Geometry: final body of the model. Coordinates: model frame, mm. Face numbers are marked on the shaded views. A direction names the side the tool comes from. Round coordinates to 2 decimals unless told otherwise and drop trailing zeros. Loops run counter-clockwise (first coordinate to the right, second up) from the corner with the lowest first, then second, coordinate; pieces in that order, holes last. Notation, with made-up numbers: M -11.5,81.5 L 33.5,81.5 A16 ccw 33.5,89.5 Z; hole C 2.5,3 d7. An arc over 180 degrees is marked long. Return JSON: item names as keys, results as strings.
from build123d import *

# Parameters (mm, degrees)
SKETCH_1_R          = 2
EXTRUDE_1_DEPTH     = 20
CUT_EXTRUDE_2_DEPTH = 14


with BuildPart() as part:
    # 草图1 → 凸台-拉伸1 (new body)
    with BuildSketch(Plane.XY):
        with BuildLine():
            Line((8.641852584, -30.917005362), (23.544151188, -8.402088166))
            Line((23.544151188, -8.402088166), (13.777542747, 27.154145307))
            ThreePointArc((13.777542747, 27.154145307), (13.313905715, 28.119907916), (12.540501442, 28.861192305))
            Line((12.540501442, 28.861192305), (8.156572048, 31.762851872))
            ThreePointArc((8.156572048, 31.762851872), (5.902657289, 32.20096852), (3.999103626, 30.917005362))
            Line((3.999103626, 30.917005362), (-23.045808654, -9.94339992))
            ThreePointArc((-23.045808654, -9.94339992), (-23.483925302, -12.197314679), (-22.199962144, -14.100868342))
            Line((-22.199962144, -14.100868342), (4.484384162, -31.762851872))
            ThreePointArc((4.484384162, -31.762851872), (6.738298922, -32.20096852), (8.641852584, -30.917005362))
        make_face()
        with Locations((6.410183267, -27.041485776)):
            Circle(SKETCH_1_R, mode=Mode.SUBTRACT)
        with Locations((17.448922973, -10.363769335)):
            Circle(SKETCH_1_R, mode=Mode.SUBTRACT)
        with Locations((-18.606391395, -10.483376217)):
            Circle(SKETCH_1_R, mode=Mode.SUBTRACT)
        with Locations((-7.567651689, 6.194340225)):
            Circle(SKETCH_1_R, mode=Mode.SUBTRACT)
        with BuildLine():
            Line((3.614616276, -20.394320576), (9.685923114, -11.221576533))
            ThreePointArc((9.685923114, -11.221576533), (9.978000879, -9.718966694), (9.122025441, -8.449930919))
            Line((9.122025441, -8.449930919), (-4.220147712, 0.381060846))
            ThreePointArc((-4.220147712, 0.381060846), (-5.722757552, 0.673138612), (-6.991793327, -0.182836827))
            Line((-6.991793327, -0.182836827), (-13.063100166, -9.35558087))
            ThreePointArc((-13.063100166, -9.35558087), (-13.355177931, -10.858190709), (-12.499202492, -12.127226485))
            Line((-12.499202492, -12.127226485), (0.842970661, -20.95821825))
            ThreePointArc((0.842970661, -20.95821825), (2.3455805, -21.250296015), (3.614616276, -20.394320576))
        make_face(mode=Mode.SUBTRACT)
        with BuildLine():
            Line((-2.181398369, 8.62528164), (12.553966944, -1.1278439))
            ThreePointArc((12.553966944, -1.1278439), (14.831422966, -1.079549075), (15.586409089, 1.069668056))
            Line((15.586409089, 1.069668056), (9.371464219, 23.695744666))
            ThreePointArc((9.371464219, 23.695744666), (7.758191259, 25.140995222), (5.775124401, 24.269878325))
            Line((5.775124401, 24.269878325), (-2.745296043, 11.396927255))
            ThreePointArc((-2.745296043, 11.396927255), (-3.037373808, 9.894317415), (-2.181398369, 8.62528164))
        make_face(mode=Mode.SUBTRACT)
    extrude(amount=EXTRUDE_1_DEPTH)

    # 草图2 → 切除-拉伸2 (cut)
    with BuildSketch(Plane.XY.offset(20)):
        Polygon((23.544151188, -8.402088166), (-8.143510051, 12.571517276), (4.702402911, 35.561922015), (37.191732114, 19.156948223), align=None)
    extrude(amount=-CUT_EXTRUDE_2_DEPTH, mode=Mode.SUBTRACT)


solid = part.part
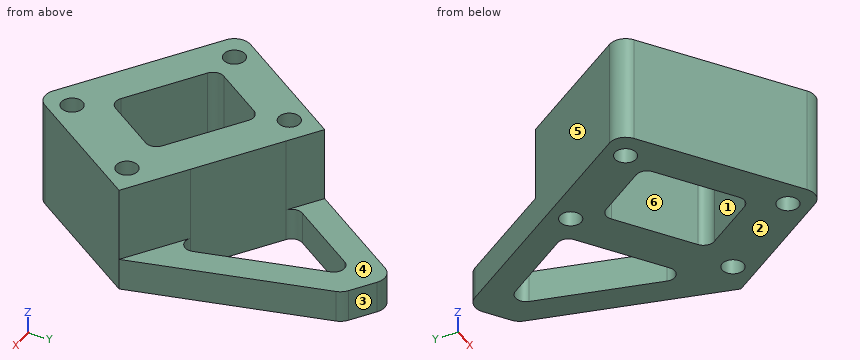
Q1. Section query C-C (z = 1.5). Output: boundary loops of the cut face in (x, y), plus the area to 3 significant figures.
Determined:
{"outline": "M -23.05,-9.94 A3 ccw -22.2,-14.1 L 4.48,-31.76 A3 ccw 8.64,-30.92 L 23.54,-8.4 L 13.78,27.15 A3 ccw 12.54,28.86 L 8.16,31.76 A3 ccw 4,30.92 Z; hole C -18.61,-10.48 d4; hole M -13.06,-9.36 A2 ccw -12.5,-12.13 L 0.84,-20.96 A2 ccw 3.61,-20.39 L 9.69,-11.22 A2 ccw 9.12,-8.45 L -4.22,0.38 A2 ccw -6.99,-0.18 Z; hole C -7.57,6.19 d4; hole M -2.75,11.4 A2 ccw -2.18,8.63 L 12.55,-1.13 A2 ccw 15.59,1.07 L 9.37,23.7 A2 ccw 5.78,24.27 Z; hole C 6.41,-27.04 d4; hole C 17.45,-10.36 d4", "area": "1,120 mm^2"}
Q2. Pull-direction query (X, two-part tool) for the marked faces 1, 2 and 3; classes: pulls with the +X half, pulls with the -X half, needs draft (parallel to the pull), parting line crosses it, or undercut.
Determined:
{"face 1": "undercut", "face 2": "needs draft", "face 3": "pulls with the +X half"}
Q3. Section query A-A (x = -11.5). Output: boundary loops of the cut face in (y, z), plus the area to 3 significant figures.
Determined:
{"outline": "M -21.18,0 L -12.79,0 L -12.79,20 L -21.18,20 Z; M -6.99,0 L 7.5,0 L 7.5,20 L -6.99,20 Z", "area": "458 mm^2"}
Q4. Section query D-D (z = 15.25). Output: boundary loops of the cut face in (x, y).
Determined:
{"outline": "M -23.05,-9.94 A3 ccw -22.2,-14.1 L 4.48,-31.76 A3 ccw 8.64,-30.92 L 23.54,-8.4 L -8.14,12.57 Z; hole C -18.61,-10.48 d4; hole M -13.06,-9.36 A2 ccw -12.5,-12.13 L 0.84,-20.96 A2 ccw 3.61,-20.39 L 9.69,-11.22 A2 ccw 9.12,-8.45 L -4.22,0.38 A2 ccw -6.99,-0.18 Z; hole C -7.57,6.19 d4; hole C 6.41,-27.04 d4; hole C 17.45,-10.36 d4"}
Q5. Pin query (flat end, axial travel): pin 1 (2 mm diameter, centred on x = 1, z = 10.5, fed in from -Y); pin 2 (1.5 mm diameter, centred on y = 4, z = 14, fed in from +X); pin 3 (4 mm diameter, centred on y = -17.5, z = 9, fed in from -X). Return the tip coordinate at first contact, or that it passes through.
Determined:
{"pin 1": "stops at y = -30.12", "pin 2": "stops at x = 5.94", "pin 3": "stops at x = -20.09"}
Q6. Material intervals for L1, parallel to Y at x = 3, z = 4.5; L2, parallel to Y at x = 5, z = 5.75; L3, parallel to X at y = 6.5, z = 5.75, sorted ascending.
Determined:
{"L1": "y = -30.78 to -20.99, -4.4 to 5.2, 20.08 to 29.41", "L2": "y = -32.04 to -28.46, -25.62 to -18.3, -5.72 to 3.87, 23.1 to 31.86", "L3": "x = -12.16 to -9.54, -5.59 to 1.03, 14.09 to 19.45"}
Q7. Section query B-B (y = -28). Output: boundary loops of the cut face in (x, z).
Determined:
{"outline": "M -1.2,0 L 4.65,0 L 4.65,20 L -1.2,20 Z; M 8.17,0 L 10.57,0 L 10.57,20 L 8.17,20 Z"}
Q8. Reachability of the marked faces 4, 5 and 6 from +Z, -Z, +X, -X, +Y, -Y: full face, straight path, thin tool, end or side. Return the list, or none.
Determined:
{"face 4": "+Z, +X, +Y", "face 5": "+Z, -Z, -X, +Y", "face 6": "+Z, -Z"}
